Geometry: final body of the model. Coordinates: model frame, mm. Face numbers are marked on the shaded views. A direction names the side the tool comes from. Coordinates: 2 decimals unless noted, no trailing zeros.
from build123d import *

# Parameters (mm, degrees)
MODEL_R             = 3
BOSS_EXTRUDE3_DEPTH = 5


with BuildPart() as part:
    # Model → Boss-Extrude3 (new body)
    with BuildSketch(Plane.YZ):
        with BuildLine():
            Line((13.23422421, -1.039678776), (14.054007268, -1.104122279))
            ThreePointArc((14.054007268, -1.104122279), (15.344427311, -0.890154011), (16.497633121, -0.272835077))
            ThreePointArc((16.497633121, -0.272835077), (16.499889045, 0), (16.497633121, 0.272835077))
            ThreePointArc((16.497633121, 0.272835077), (15.34442594, 0.890147785), (14.054007268, 1.104113746))
            Line((14.054007268, 1.104113746), (13.23422421, 1.039678776))
            ThreePointArc((13.23422421, 1.039678776), (13.111569145, 2.076626337), (12.907793057, 3.100725851))
            Line((12.907793057, 3.100725851), (13.707329207, 3.292922702))
            ThreePointArc((13.707329207, 3.292922702), (14.868425654, 3.895152548), (15.774406226, 4.838563885))
            ThreePointArc((15.774406226, 4.838563885), (15.692222832, 5.098794143), (15.60574669, 5.357629562))
            ThreePointArc((15.60574669, 5.357629562), (14.318274111, 5.588337046), (13.024951323, 5.393073752))
            Line((13.024951323, 5.393073752), (12.265239884, 5.078337619))
            ThreePointArc((12.265239884, 5.078337619), (11.828111536, 6.02672381), (11.317788592, 6.937815491))
            Line((11.317788592, 6.937815491), (12.018874896, 7.367617174))
            ThreePointArc((12.018874896, 7.367617174), (12.937059572, 8.29919163), (13.507168648, 9.476421305))
            ThreePointArc((13.507168648, 9.476421305), (13.348651089, 9.698493941), (13.186482736, 9.917914762))
            ThreePointArc((13.186482736, 9.917914762), (11.890651127, 9.739508353), (10.72089422, 9.154121999))
            Line((10.72089422, 9.154121999), (10.095695669, 8.619892769))
            ThreePointArc((10.095695669, 8.619892769), (9.386972883, 9.386712017), (8.620173331, 10.095456114))
            Line((8.620173331, 10.095456114), (9.153880493, 10.721137246))
            ThreePointArc((9.153880493, 10.721137246), (9.739259724, 11.890873647), (9.917672889, 13.186682597))
            ThreePointArc((9.917672889, 13.186682597), (9.698234401, 13.348871345), (9.476143545, 13.507408695))
            ThreePointArc((9.476143545, 13.507408695), (8.298924763, 12.937292239), (7.367360076, 12.019107034))
            Line((7.367360076, 12.019107034), (6.937941159, 11.317711556))
            ThreePointArc((6.937941159, 11.317711556), (6.026818359, 11.828063361), (5.078397518, 12.265215084))
            Line((5.078397518, 12.265215084), (5.393131966, 13.025188132))
            ThreePointArc((5.393131966, 13.025188132), (5.588395055, 14.318515258), (5.357684148, 15.605991551))
            ThreePointArc((5.357684148, 15.605991551), (5.098848094, 15.692468837), (4.838617177, 15.774653351))
            ThreePointArc((4.838617177, 15.774653351), (3.895206219, 14.868670943), (3.292977313, 13.707572882))
            Line((3.292977313, 13.707572882), (3.100760275, 12.907784787))
            ThreePointArc((3.100760275, 12.907784787), (2.076645901, 13.111566047), (1.039682977, 13.23422388))
            Line((1.039682977, 13.23422388), (1.104104268, 14.054249317))
            ThreePointArc((1.104104268, 14.054249317), (0.890123262, 15.344688358), (0.272780986, 16.497905294))
            ThreePointArc((0.272780986, 16.497905294), (0, 16.500160321), (-0.272780986, 16.497905294))
            ThreePointArc((-0.272780986, 16.497905294), (-0.890123262, 15.344688358), (-1.104104268, 14.054249317))
            Line((-1.104104268, 14.054249317), (-1.039682977, 13.23422388))
            ThreePointArc((-1.039682977, 13.23422388), (-2.076645901, 13.111566047), (-3.100760275, 12.907784787))
            Line((-3.100760275, 12.907784787), (-3.292901189, 13.707572882))
            ThreePointArc((-3.292901189, 13.707572882), (-3.895130728, 14.8686712), (-4.838542654, 15.774653351))
            ThreePointArc((-4.838542654, 15.774653351), (-5.09877719, 15.692468897), (-5.357616845, 15.605991551))
            ThreePointArc((-5.357616845, 15.605991551), (-5.588327412, 14.318515249), (-5.393064608, 13.025188132))
            Line((-5.393064608, 13.025188132), (-5.078397518, 12.265215084))
            ThreePointArc((-5.078397518, 12.265215084), (-6.026818359, 11.828063361), (-6.937941159, 11.317711556))
            Line((-6.937941159, 11.317711556), (-7.367917741, 12.019107034))
            ThreePointArc((-7.367917741, 12.019107034), (-8.299522933, 12.93730687), (-9.476792265, 13.507408695))
            ThreePointArc((-9.476792265, 13.507408695), (-9.69882033, 13.348870312), (-9.918196776, 13.186682597))
            ThreePointArc((-9.918196776, 13.186682597), (-9.739783579, 11.890873626), (-9.154404251, 10.721137246))
            Line((-9.154404251, 10.721137246), (-8.620173331, 10.095456114))
            ThreePointArc((-8.620173331, 10.095456114), (-9.386972883, 9.386712017), (-10.095695669, 8.619892769))
            Line((-10.095695669, 8.619892769), (-10.721421894, 9.154121999))
            ThreePointArc((-10.721421894, 9.154121999), (-11.891119242, 9.739488239), (-13.18688523, 9.917914762))
            ThreePointArc((-13.18688523, 9.917914762), (-13.349106741, 9.698494383), (-13.507677449, 9.476421305))
            ThreePointArc((-13.507677449, 9.476421305), (-12.937567793, 8.29919139), (-12.019382207, 7.367617174))
            Line((-12.019382207, 7.367617174), (-11.317788592, 6.937815491))
            ThreePointArc((-11.317788592, 6.937815491), (-11.828111536, 6.02672381), (-12.265239884, 5.078337619))
            Line((-12.265239884, 5.078337619), (-13.025469237, 5.393073752))
            ThreePointArc((-13.025469237, 5.393073752), (-14.318795833, 5.588338267), (-15.606272205, 5.357629562))
            ThreePointArc((-15.606272205, 5.357629562), (-15.692748124, 5.098794139), (-15.774931305, 4.838563885))
            ThreePointArc((-15.774931305, 4.838563885), (-14.868950755, 3.895152556), (-13.707854335, 3.292922702))
            Line((-13.707854335, 3.292922702), (-12.907793057, 3.100725851))
            ThreePointArc((-12.907793057, 3.100725851), (-13.111569145, 2.076626337), (-13.23422421, 1.039678776))
            Line((-13.23422421, 1.039678776), (-14.05453238, 1.104113746))
            ThreePointArc((-14.05453238, 1.104113746), (-15.344937836, 0.890143752), (-16.498133136, 0.272835077))
            ThreePointArc((-16.498133136, 0.272835077), (-16.500389058, 0), (-16.498133136, -0.272835077))
            ThreePointArc((-16.498133136, -0.272835077), (-15.344939207, -0.890149979), (-14.05453238, -1.104122279))
            Line((-14.05453238, -1.104122279), (-13.23422421, -1.039678776))
            ThreePointArc((-13.23422421, -1.039678776), (-13.111569145, -2.076626337), (-12.907793057, -3.100725851))
            Line((-12.907793057, -3.100725851), (-13.707854335, -3.292963653))
            ThreePointArc((-13.707854335, -3.292963653), (-14.868950761, -3.895193523), (-15.774931305, -4.838604875))
            ThreePointArc((-15.774931305, -4.838604875), (-15.692748091, -5.098833138), (-15.606272205, -5.35766658))
            ThreePointArc((-15.606272205, -5.35766658), (-14.318795843, -5.588375668), (-13.025469237, -5.393110833))
            Line((-13.025469237, -5.393110833), (-12.265239884, -5.078337619))
            ThreePointArc((-12.265239884, -5.078337619), (-11.828111536, -6.02672381), (-11.317788592, -6.937815491))
            Line((-11.317788592, -6.937815491), (-12.019382207, -7.367660494))
            ThreePointArc((-12.019382207, -7.367660494), (-12.937567956, -8.299235159), (-13.507677449, -9.476465634))
            ThreePointArc((-13.507677449, -9.476465634), (-13.34910671, -9.698536821), (-13.18688523, -9.917955332))
            ThreePointArc((-13.18688523, -9.917955332), (-11.891119181, -9.739528715), (-10.721421894, -9.154162191))
            Line((-10.721421894, -9.154162191), (-10.095695669, -8.619892769))
            ThreePointArc((-10.095695669, -8.619892769), (-9.386972883, -9.386712017), (-8.620173331, -10.095456114))
            Line((-8.620173331, -10.095456114), (-9.154404251, -10.721178465))
            ThreePointArc((-9.154404251, -10.721178465), (-9.739783866, -11.890915694), (-9.918196776, -13.186725599))
            ThreePointArc((-9.918196776, -13.186725599), (-9.698820328, -13.348913221), (-9.476792265, -13.507451513))
            ThreePointArc((-9.476792265, -13.507451513), (-8.299522952, -12.937349732), (-7.367917741, -12.019149967))
            Line((-7.367917741, -12.019149967), (-6.937941159, -11.317711556))
            ThreePointArc((-6.937941159, -11.317711556), (-6.026818359, -11.828063361), (-5.078397518, -12.265215084))
            Line((-5.078397518, -12.265215084), (-5.393064608, -13.025228542))
            ThreePointArc((-5.393064608, -13.025228542), (-5.588327412, -14.31855566), (-5.357616845, -15.606031962))
            ThreePointArc((-5.357616845, -15.606031962), (-5.098777189, -15.692509269), (-4.838542654, -15.774693688))
            ThreePointArc((-4.838542654, -15.774693688), (-3.895130728, -14.868711537), (-3.292901189, -13.707613219))
            Line((-3.292901189, -13.707613219), (-3.100760275, -12.907784787))
            ThreePointArc((-3.100760275, -12.907784787), (-2.076645901, -13.111566047), (-1.039682977, -13.23422388))
            Line((-1.039682977, -13.23422388), (-1.104104268, -14.054290311))
            ThreePointArc((-1.104104268, -14.054290311), (-0.890123262, -15.344729352), (-0.272780986, -16.497946289))
            ThreePointArc((-0.272780986, -16.497946289), (0, -16.500201314), (0.272780986, -16.497946289))
            ThreePointArc((0.272780986, -16.497946289), (0.890123262, -15.344729352), (1.104104268, -14.054290311))
            Line((1.104104268, -14.054290311), (1.039682977, -13.23422388))
            ThreePointArc((1.039682977, -13.23422388), (2.076645901, -13.111566047), (3.100760275, -12.907784787))
            Line((3.100760275, -12.907784787), (3.292977313, -13.707613219))
            ThreePointArc((3.292977313, -13.707613219), (3.895206219, -14.868711279), (4.838617177, -15.774693688))
            ThreePointArc((4.838617177, -15.774693688), (5.098848093, -15.69250921), (5.357684148, -15.606031962))
            ThreePointArc((5.357684148, -15.606031962), (5.588395055, -14.318555669), (5.393131966, -13.025228542))
            Line((5.393131966, -13.025228542), (5.078397518, -12.265215084))
            ThreePointArc((5.078397518, -12.265215084), (6.026818359, -11.828063361), (6.937941159, -11.317711556))
            Line((6.937941159, -11.317711556), (7.367360076, -12.019149967))
            ThreePointArc((7.367360076, -12.019149967), (8.298924781, -12.937335102), (9.476143545, -13.507451513))
            ThreePointArc((9.476143545, -13.507451513), (9.698234399, -13.348914253), (9.917672889, -13.186725599))
            ThreePointArc((9.917672889, -13.186725599), (9.73926001, -11.890915714), (9.153880493, -10.721178465))
            Line((9.153880493, -10.721178465), (8.620173331, -10.095456114))
            ThreePointArc((8.620173331, -10.095456114), (9.386972883, -9.386712017), (10.095695669, -8.619892769))
            Line((10.095695669, -8.619892769), (10.72089422, -9.154162191))
            ThreePointArc((10.72089422, -9.154162191), (11.890651066, -9.739548829), (13.186482736, -9.917955332))
            ThreePointArc((13.186482736, -9.917955332), (13.348651058, -9.698536379), (13.507168648, -9.476465634))
            ThreePointArc((13.507168648, -9.476465634), (12.937059735, -8.299235399), (12.018874896, -7.367660494))
            Line((12.018874896, -7.367660494), (11.317788592, -6.937815491))
            ThreePointArc((11.317788592, -6.937815491), (11.828111536, -6.02672381), (12.265239884, -5.078337619))
            Line((12.265239884, -5.078337619), (13.024951323, -5.393110833))
            ThreePointArc((13.024951323, -5.393110833), (14.318274121, -5.588374447), (15.60574669, -5.35766658))
            ThreePointArc((15.60574669, -5.35766658), (15.692222799, -5.098833142), (15.774406226, -4.838604875))
            ThreePointArc((15.774406226, -4.838604875), (14.86842566, -3.895193515), (13.707329207, -3.292963653))
            Line((13.707329207, -3.292963653), (12.907793057, -3.100725851))
            ThreePointArc((12.907793057, -3.100725851), (13.111569145, -2.076626337), (13.23422421, -1.039678776))
        make_face()
        with Locations(Location((0, 0, 0), (0, 0, 270))):
            Circle(MODEL_R, mode=Mode.SUBTRACT)
    extrude(amount=BOSS_EXTRUDE3_DEPTH)


solid = part.part
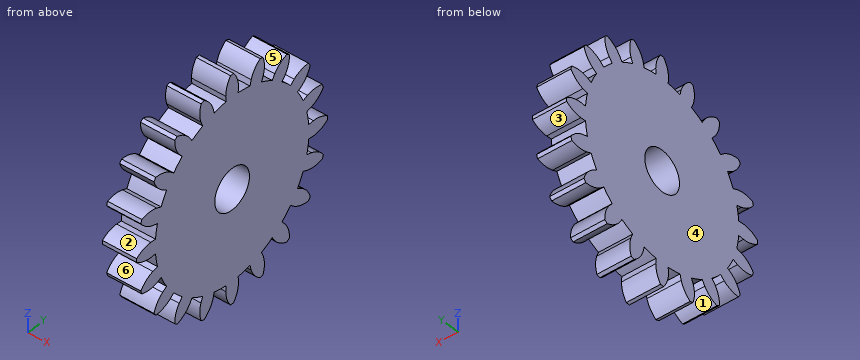
Item 1: Material intervals for probe 1 along Y at (x, z) = (2.6, 0); probe 2 along Z at (x, y) = (1.5, -14); probe 3 along Z at (x, y) = (3.4, 14.5), sorted ascending.
Derived:
probe 1: y = -16.5 to -3, 3 to 16.5
probe 2: z = -5.58 to -3.4, -1.1 to 1.1, 3.4 to 5.58
probe 3: z = -5.58 to -3.65, -1.08 to 1.08, 3.65 to 5.58
Item 2: Pin query (flat end, axial travel): pin 1 (5 mm diameter, centred on y = 0, z = 0, fed in from +X); pin 2 (2 mm diameter, centred on x = 2, y = -4.5, fed in from +Z); pin 3 (3 mm diameter, centred on x = 3, z = 7.5, fed in from -Y); pin 4 (1.5 mm diameter, centred on x = 1, z = 7.5, fed in from +Y). Return the tip coordinate at first contact, or that it passes through.
Derived:
pin 1: passes through
pin 2: stops at z = 15.77
pin 3: stops at y = -13.33
pin 4: stops at y = 12.9
Item 3: Pull-direction query (Y, two-part tool) for the marked faces 4, 5 and 6; classes: released by +Y, released by -Y, zero draft, split by the parting line, or undercut.
Derived:
face 4: zero draft
face 5: undercut
face 6: released by -Y
Item 4: Set-up query: the marked faces 1, 2 and 3. Return all of +Z, -Z, +X, -X, +Y, -Y with unobstructed straight access to the full face (end or side cutting, diameter ignored); none if empty.
Derived:
face 1: -Z, +X, -X
face 2: +X, -X, -Y
face 3: +X, -X, +Y
